from build123d import *

# Parameters (mm, degrees)
SKETCH1_W           = 240
SKETCH1_H           = 240
SKETCH1_W_2         = 30
SKETCH1_H_2         = 5
SKETCH1_W_3         = 5
SKETCH1_H_3         = 30
BOSS_EXTRUDE1_DEPTH = 5


with BuildPart() as part:
    # Sketch1 → Boss-Extrude1 (new body)
    with BuildSketch(Plane.XY):
        Rectangle(SKETCH1_W, SKETCH1_H)
        with Locations((0, 122.5)):
            Rectangle(SKETCH1_W_2, SKETCH1_H_2)
        with Locations((95, 122.5)):
            Rectangle(SKETCH1_W_2, SKETCH1_H_2)
        with Locations((-122.5, 95)):
            Rectangle(SKETCH1_W_3, SKETCH1_H_3)
        with Locations((-122.5, 0)):
            Rectangle(SKETCH1_W_3, SKETCH1_H_3)
        with Locations((-122.5, -95)):
            Rectangle(SKETCH1_W_3, SKETCH1_H_3)
        with Locations((-95, -122.5)):
            Rectangle(SKETCH1_W_2, SKETCH1_H_2)
        with Locations((0, -122.5)):
            Rectangle(SKETCH1_W_2, SKETCH1_H_2)
        with Locations((95, -122.5)):
            Rectangle(SKETCH1_W_2, SKETCH1_H_2)
        with Locations((122.5, -95)):
            Rectangle(SKETCH1_W_3, SKETCH1_H_3)
        with Locations((122.5, 0)):
            Rectangle(SKETCH1_W_3, SKETCH1_H_3)
        with Locations((122.5, 95)):
            Rectangle(SKETCH1_W_3, SKETCH1_H_3)
        with Locations((-95, 122.5)):
            Rectangle(SKETCH1_W_2, SKETCH1_H_2)
    extrude(amount=BOSS_EXTRUDE1_DEPTH)


solid = part.part
Work out the finished part from the listing and answer in its coordinate system (mm). Coordinates: 2 decimals unless noted, no trailing zeros. Write each loop counter-clockwise with the first axis right and the second up, starting at its lowest first coordinate (ties: lowest second). Pieces come first, ordered by that corner, then holes. Notation, with made-up numbers: M 27,35 L 48,35 A13 cw 48,41 Z; hole C 61.25,47 d9. An arc over 180 degrees is marked long. Answer as CSV lines item,"result". Start each with the question number.
Item 1: Consider L1, parallel to X at y = 24, z = 1. Determine where the line is inside the solid, lowest interval first.
Item 2: Flat-ended cylindrical pins translate along their axes: P1, Ø1.5, axis at x = -121.5, z = 3.5, coming from the -Y side; P2, Ø2.5, axis at x = -121.5, z = 2.5, coming from the +Y side; P3, Ø1.5, axis at y = 31.5, z = 3.5, coming from the -X side. Find the tip coordinate at first contact, or state that the pin passes through.
Item 3: Section A-A on y = 50 is taken. Write down the section's boundary in (x, z).
Checks:
1,L1,"x = -120 to 120"
2,P1,"stops at y = -110"
2,P2,"stops at y = 110"
2,P3,"stops at x = -120"
3,outline,"M -120,0 L 120,0 L 120,5 L -120,5 Z"
